from build123d import *

# Parameters (mm, degrees)
PLATE_DEPTH         = 9
SKETCH3_R           = 1.6
HEX_HOLES_DEPTH     = 128.597021909
SKETCH4_R           = 1.6
ARDUINO_HOLES_DEPTH = 128.597021909
SKETCH5_W           = 40
SKETCH5_H           = 100
CUT_EXTRUDE1_DEPTH  = 128.597021909
FILLET1_R           = 10


with BuildPart() as part:
    # Sketch1 → Plate (new body)
    with BuildSketch(Plane(origin=(0, 0, 0), x_dir=(1, 0, 0), z_dir=(0, 1, 0))):
        with BuildLine():
            Line((-65, -90), (65, -90))
            ThreePointArc((65, -90), (82.67766953, -82.67766953), (90, -65))
            Line((90, -65), (90, 65))
            ThreePointArc((90, 65), (82.67766953, 82.67766953), (65, 90))
            Line((65, 90), (-65, 90))
            ThreePointArc((-65, 90), (-82.67766953, 82.67766953), (-90, 65))
            Line((-90, 65), (-90, -65))
            ThreePointArc((-90, -65), (-82.67766953, -82.67766953), (-65, -90))
        make_face()
    extrude(amount=PLATE_DEPTH)

    # Sketch3 → Hex Holes (cut, through all)
    with BuildSketch(Plane(origin=(0, 9, 0), x_dir=(1, 0, 0), z_dir=(0, 1, 0))):
        with Locations(Location((-65, 80, 0), (0, 0, 270))):
            Circle(SKETCH3_R)
        with Locations(Location((-80, 65, 0), (0, 0, 270))):
            Circle(SKETCH3_R)
        with Locations(Location((80, 65, 0), (0, 0, 270))):
            Circle(SKETCH3_R)
        with Locations(Location((80, -65, 0), (0, 0, 270))):
            Circle(SKETCH3_R)
        with Locations(Location((65, 80, 0), (0, 0, 270))):
            Circle(SKETCH3_R)
        with Locations(Location((65, -80, 0), (0, 0, 270))):
            Circle(SKETCH3_R)
        with Locations(Location((-65, -80, 0), (0, 0, 270))):
            Circle(SKETCH3_R)
        with Locations(Location((-80, -65, 0), (0, 0, 270))):
            Circle(SKETCH3_R)
    extrude(amount=-HEX_HOLES_DEPTH, mode=Mode.SUBTRACT)

    # Sketch4 → Arduino Holes (cut, through all)
    with BuildSketch(Plane(origin=(0, 9, 0), x_dir=(1, 0, 0), z_dir=(0, 1, 0))):
        with Locations(Location((-24.5, -31, 0), (0, 0, 270))):
            Circle(SKETCH4_R)
        with Locations(Location((24.5, -31, 0), (0, 0, 270))):
            Circle(SKETCH4_R)
        with Locations(Location((-19.25, 31, 0), (0, 0, 270))):
            Circle(SKETCH4_R)
        with Locations(Location((19.25, 31, 0), (0, 0, 270))):
            Circle(SKETCH4_R)
    extrude(amount=-ARDUINO_HOLES_DEPTH, mode=Mode.SUBTRACT)

    # Sketch5 → Cut-Extrude1 (cut, through all)
    with BuildSketch(Plane(origin=(0, 9, 0), x_dir=(1, 0, 0), z_dir=(0, 1, 0))):
        with Locations((-70, 0)):
            Rectangle(SKETCH5_W, SKETCH5_H)
        with Locations((70, 0)):
            Rectangle(SKETCH5_W, SKETCH5_H)
    extrude(amount=-CUT_EXTRUDE1_DEPTH, mode=Mode.SUBTRACT)

    # Fillet1
    fillet1_edges = [part.edges().sort_by_distance(p)[0] for p in [
        (50, 4.5, 50),
        (50, 4.5, -50),
        (-50, 4.5, -50),
        (-50, 4.5, 50),
    ]]
    fillet(fillet1_edges, radius=FILLET1_R)


solid = part.part
The listing builds one solid part. Answer for the finished solid, in the listing's coordinates (mm). A direction names the side the tool comes from. Coordinates: 2 decimals unless noted, no trailing zeros. Write each loop counter-clockwise with the first axis right and the second up, starting at its lowest first coordinate (ties: lowest second). Pieces come first, ordered by that corner, then holes. Notation, with made-up numbers: (23, 52.25) -> (53, 52.25) arc R25 cw to (53, 80.25) -> close; hole circle Ø7 at (-27, 84.25). An arc over 180 degrees is marked (long way). One line per question, with ' | ' between items.
1. Section B-B (z = 16.5) is taken. Determine the outline of the cut face in (x, y), and give its area (3 significant figures).
Verdict:
outline: (-50, 0) -> (50, 0) -> (50, 9) -> (-50, 9) -> close | area: 900 mm^2
2. Section A-A (y = 5) is taken. State how many separate pieces and enclosed holes the cut face has, and give its area (3 significant figures).
Verdict:
separate pieces: 1 | enclosed holes: 12 | area: 23,900 mm^2
3. Which of the six approach directions +Z, -Z, +X, -X, +Y, -Y give full straight-line access (tool end or side, diameter ignored) to faces 5 (the cylindrical face through (-82.482, 4.437, -82.871)), 6 (the flat face through (75, 5, 50)), 7 (the cylindrical face through (-52.85, 4.44, -46.99))?
Verdict:
face 5: -Z, -X, +Y, -Y | face 6: +X, +Y, -Y | face 7: -X, +Y, -Y
4. Straight lines are drawn through the part: line 1 (X direction, y = 3.75, z = 65); line 2 (X direction, y = 6, z = 31); line 3 (Z direction, x = -65, y = 2.5). For each, find the intervals that lie inside material, in ascending order.
Verdict:
line 1: x = -90 to -81.6, -78.4 to 78.4, 81.6 to 90 | line 2: x = -50 to -26.1, -22.9 to 22.9, 26.1 to 50 | line 3: z = -90 to -81.6, -78.4 to -50, 50 to 78.4, 81.6 to 90
5. For a pull along Z with two mould halves and no side action, classify faces 1 (the cylindrical face through (-82.871, 4.437, 82.482)), 2 (the flat face through (-75, 5, -50)), 3 (the flat face through (-1, 9, -1)), 4 (the cylindrical face through (82.871, 4.437, -82.482)) as released by +Z, released by -Z, zero draft, split by the parting line, or undercut.
Verdict:
face 1: released by +Z | face 2: undercut | face 3: zero draft | face 4: released by -Z
6. Given pin 1 Ø3 at (x, z) = (19.25, -31) entering from +Y; pin 2 Ø2.5 at (y, z) = (4, 0) entering from -X; pin 3 Ø4.5 at (x, y) = (71.5, 3) entering from -Z; pin 4 Ø1.5 at (x, y) = (-70.5, 2) entering from -Z, each flat-ended and moving along its own axis, determine where each tip first touches the part or whether it passes through.
Verdict:
pin 1: passes through | pin 2: stops at x = -50 | pin 3: stops at z = -89.64 | pin 4: stops at z = -89.54
